Input: part model. Units: mm. Frame: model coordinates. A direction names the side the tool comes from. Round coordinates to 2 decimals unless told otherwise and drop trailing zeros. Loops run counter-clockwise (first coordinate to the right, second up) from the corner with the lowest first, then second, coordinate; pieces in that order, holes last.
1) Ray query, line 1 along X through (y, z) = (-17, 2.5); line 2 along X through (y, z) = (-1.5, 1.25); line 3 along Y through (x, z) = (-41, 3.25). Return the intervals inside material, ascending.
2) Section A-A, the plane x = 54. Return loops of the section in (y, z), and give its area (3 significant figures).
3) Access query for faces 1 (the face through (39, -11, 3)), 2 (the face through (58.643, -33, 3)), 3 (the face through (-61.357, -33, 3)). Directions: +Z, -Z, +X, -X, +Y, -Y. A direction counts if a zero-diameter tool reaches every point of the face in a straight line with its end or side. Return the directions, or none.
4) Section C-C, the plane z = 1. State how many separate pieces and enclosed holes the cut face has, and give its area (3 significant figures).
5) Section B-B, the plane y = -32. Return loops of the section in (x, z).
6) Draft query along X for faces 4 (the face through (-41, -11, 3)), 5 (the face through (102.94, 3.986, 3.159)), 6 (the face through (93, -30, 3)). Return one class per face: pulls with the +X half, pulls with the -X half, needs draft (parallel to the pull), parting line crosses it, or undercut.
7) First-contact query: pin 1 (1 mm diameter, centred on y = -14, z = 5.5, fed in from -X); pin 2 (3 mm diameter, centred on y = -32, z = 4, fed in from +X); pin 3 (3 mm diameter, centred on y = 4.5, z = 5.5, fed in from -X); pin 4 (4 mm diameter, centred on x = -49, y = -3.5, fed in from +Z). Flat tips, straight axial feed; report the tip coordinate or a pass-through.
from build123d import *

# Parameters (mm, degrees)
F0_W     = 20
F0_H     = 6.35
F1_DEPTH = 6.35
F2_R     = 2


with BuildPart() as f1:
    # F0 (on Top) → F1 (new body)
    with BuildSketch(Plane.XY):
        with BuildLine():
            Line((88.642785, 10), (-71.357215, 10))
            ThreePointArc((-71.357215, 10), (-85.49935, 4.142136), (-91.357215, -10))
            Line((-91.357215, -10), (-91.357215, -30))
            Line((-91.357215, -30), (-61.357215, -30))
            Line((-61.357215, -30), (-41.357215, -30))
            Line((-41.357215, -30), (58.642785, -30))
            Line((58.642785, -30), (78.642785, -30))
            Line((78.642785, -30), (108.642785, -30))
            Line((108.642785, -30), (108.642785, -10))
            ThreePointArc((108.642785, -10), (102.784921, 4.142136), (88.642785, 10))
        make_face()
        with Locations((-41.357215, -14.175)):
            Rectangle(F0_W, F0_H, mode=Mode.SUBTRACT)
        with Locations((38.642785, -14.175)):
            Rectangle(F0_W, F0_H, mode=Mode.SUBTRACT)
        with BuildLine():
            ThreePointArc((-71.357215, -10), (-76.357215, -5), (-71.357215, 0))
            Line((-71.357215, 0), (78.642785, 0))
            ThreePointArc((78.642785, 0), (82.178319, -1.464466), (83.642785, -5))
            ThreePointArc((83.642785, -5), (82.178319, -8.535534), (78.642785, -10))
            Line((78.642785, -10), (-71.357215, -10))
        make_face(mode=Mode.SUBTRACT)
        with BuildLine():
            Line((97.292785, -15), (97.292785, 0))
            Line((97.292785, 0), (98.642785, 0))
            ThreePointArc((98.642785, 0), (102.178319, -1.464466), (103.642785, -5))
            Line((103.642785, -5), (103.642785, -15))
            Line((103.642785, -15), (97.292785, -15))
        make_face(mode=Mode.SUBTRACT)
        with Locations((-51.357215, -33.175)):
            Rectangle(F0_W, F0_H)
        with Locations((68.642785, -33.175)):
            Rectangle(F0_W, F0_H)
    extrude(amount=F1_DEPTH)

    # F2
    f2_edges = [f1.edges().sort_by_distance(p)[0] for p in [
        (-85.49935, 4.142136, 6.35),
        (8.642785, 10, 0),
        (-51.357215, -36.35, 0),
        (68.642785, -36.35, 0),
    ]]
    fillet(f2_edges, radius=F2_R)


solid = f1.part
Final values:
1. line 1: x = -91.36 to -51.36, -31.36 to 28.64, 48.64 to 108.64
1. line 2: x = -89.3 to -74.93, 82.21 to 97.29, 102.21 to 106.59
1. line 3: y = -30 to -17.35, -11 to -10, 0 to 10
2. outline: (-30, 0) - (-10, 0) - (-10, 6.35) - (-30, 6.35) - close; (0, 0) - (8, 0) arc R2 ccw to (10, 2) - (10, 4.35) arc R2 ccw to (8, 6.35) - (0, 6.35) - close
2. area: 189 mm2
3. face 1: +Z, -Z
3. face 2: +Z, -Z, -Y
3. face 3: +Z, -Z, -X, -Y
4. separate pieces: 1
4. enclosed holes: 4
4. area: 6,080 mm2
5. outline: (-61.36, 0) - (-41.36, 0) - (-41.36, 6.35) - (-61.36, 6.35) - close; (58.64, 0) - (78.64, 0) - (78.64, 6.35) - (58.64, 6.35) - close
6. face 4: undercut
6. face 5: pulls with the +X half
6. face 6: needs draft
7. pin 1: stops at x = -91.25
7. pin 2: stops at x = 78.64
7. pin 3: stops at x = -86.35
7. pin 4: passes through
